Geometry check sheet. Reference: the model listing, model coordinates, mm. A direction names the side the tool comes from. Coordinates: 2 decimals unless noted, no trailing zeros. Loops run counter-clockwise (first coordinate to the right, second up) from the corner with the lowest first, then second, coordinate; pieces in that order, holes last. Notation, with made-up numbers: (-9.75, 82.25) - (0.25, 82.25) arc R26 ccw to (0.25, 118.25) - close; hole circle Ø10 at (75.25, 37.25). An arc over 180 degrees is marked (long way). Write each question's results on one line, items separated by ' | '. Start each with the question number.
(1) Sectioned sample at A-A (x = -16). Enter the section's corners in (y, z).
(2) Sectioned sample at C-C (x = -8.5). Enter the section's corners in (y, z), plus the area to 3 significant figures.
(3) Sectioned sample at B-B (z = 0.25). State how many separate pieces and enclosed holes the cut face has, plus the area to 3 significant figures.
(4) Material ranges on probe 1 along Y at (x, z) = (-19, 0.1); probe 2 along Y at (x, z) = (-10, 0.5); probe 3 along X at (y, z) = (3, 0.2), recorded low to high.
(5) Mould release check, pull along X, two halves, no side actions. Record for faces 3 (the face through (-10, 2, 0.8)), 4 (the face through (-8.82, 7.37, 0.41)), 5 (the face through (1.906, 13.278, 0.394)): pulls with the +X half, pulls with the -X half, needs draft (parallel to the pull), parting line crosses it, or undercut.
(6) Sectioned sample at D-D (y = 3). Enter the section's corners in (x, z), plus the area to 3 significant figures.
(7) Access from +Z, -Z, +X, -X, +Y, -Y to the whole of each face (thin tool, end or side, straight path). Record for faces 1 (the face through (1.906, -14.722, 0.394)), 2 (the face through (-8.865, 3.125, 0.406)).
from build123d import *

# Parameters (mm, degrees)
F0_W     = 32
F0_H     = 38
F1_DEPTH = 0.8
F2_R     = 1
F2_W     = 18
F2_H     = 6
F3_DEPTH = 0.8
F4_R     = 2.99999


# Not quite as in the source:
# - a fillet or chamfer is up to 0.001 mm smaller than in the source, because OpenCascade refuses the exact size


with BuildPart() as f1:
    # F0 (on Top) → F1 (new body)
    with BuildSketch(Plane.XY):
        with Locations((-9.963327945, 1.2697370127)):
            Rectangle(F0_W, F0_H)
    extrude(amount=F1_DEPTH)

    # F2 (on face) → F3 (cut, through all)
    with BuildSketch(Plane(origin=(0, 0, 0), x_dir=(1, 0, 0), z_dir=(0, 0, -1))):
        with Locations((-23.463327945, 13.7302629873)):
            Circle(F2_R)
        with Locations((-23.463327945, -14.2697370127)):
            Circle(F2_R)
        with Locations((2.036672055, 13.7302629873)):
            Circle(F2_R)
        with Locations((2.036672055, -14.2697370127)):
            Circle(F2_R)
        with Locations((-16.963327945, -5.2697370127)):
            Rectangle(F2_W, F2_H)
    extrude(amount=-F3_DEPTH, mode=Mode.SUBTRACT)

    # F4 (radius 3 in the source; OpenCascade refuses exactly that, so slightly less here)
    f4_edges = [f1.edges().sort_by_distance(p)[0] for p in [
        (-7.963328, 8.269737, 0.4),
        (-7.963328, 2.269737, 0.4),
    ]]
    fillet(f4_edges, radius=F4_R)


solid = f1.part
Outcome:
1) outline: (-17.73, 0) - (2.27, 0) - (2.27, 0.8) - (-17.73, 0.8) - close; (8.27, 0) - (20.27, 0) - (20.27, 0.8) - (8.27, 0.8) - close
2) outline: (-17.73, 0) - (3.56, 0) - (3.56, 0.8) - (-17.73, 0.8) - close; (6.98, 0) - (20.27, 0) - (20.27, 0.8) - (6.98, 0.8) - close | area: 27.7 mm2
3) separate pieces: 1 | enclosed holes: 4 | area: 1,100 mm2
4) probe 1: y = -17.73 to 2.27, 8.27 to 20.27 | probe 2: y = -17.73 to 2.43, 8.11 to 20.27 | probe 3: x = -9 to 6.04
5) face 3: needs draft | face 4: pulls with the -X half | face 5: undercut
6) outline: (-9, 0) - (6.04, 0) - (6.04, 0.8) - (-9, 0.8) - close | area: 12.0 mm2
7) face 1: +Z, -Z | face 2: +Z, -Z, -X
